Autodesk Fusion 360 part; units mm, degrees
sketch "Sketch1" plane through (0, 0, 0) normal (0, 0, 1) x (1, 0, 0)
  circle A0 centre (0, 0) radius 9.5
  line L0 (12, 5) -> (-12, 5)
  line L1 (-12, 5) -> (-12, -5)
  line L2 (-12, -5) -> (12, -5)
  line L3 (12, -5) -> (12, 5)
  line L4 (-12, -5) -> (-22, -5)
  line L5 (-22, -5) -> (-22, 5)
  line L6 (-22, 5) -> (-12, 5)
  line L7 (-12, 5) -> (-12, -5)
  line L8 (12, -5) -> (22, -5)
  line L9 (22, -5) -> (22, 5)
  line L10 (22, 5) -> (12, 5)
  line L11 (12, 5) -> (12, -5)
  circle A1 centre (17, 0) radius 1.825
  circle A2 centre (-17, 0) radius 1.825
  dimension "d1" = 19
  dimension "d2" = 5
  dimension "d3" = 5
  dimension "d4" = 12
  dimension "d19" = 24
  dimension "d20" = 3.65
  dimension "d21" = 3.65
extrude "Extrude1" add sketch "Sketch1" along normal blind 3 contours A0 L0 L2 L3 L11 | A0 L0 L1 L2 L7 makes body 1 at (-9.0078, 3.0183, 2) makes body 2 at (8.3, 4.6217, 2)
extrude "Extrude2" add sketch "Sketch1" along normal blind 13.5 contours A0 L0 L2 | A0 L0 | A0 L2 bodies 1 2
sketch "Sketch2" plane through (0, 0, 0) normal (0, 1, 0) x (1, 0, 0)
  line L0 (-9.5, -15) -> (9.5, -15)
  line L1 (9.5, -15) -> (9.5, 0)
  line L2 (9.5, 0) -> (-9.5, 0)
  line L3 (-9.5, 0) -> (-9.5, -15)
  line L4 (9.5, 0) -> (-9.5, 0)
  line L5 (-9.5, 0) -> (-9.5, -3)
  line L6 (-9.5, -3) -> (9.5, -3)
  line L7 (9.5, -3) -> (9.5, 0)
  line L8 (-9.5, -15) -> (9.5, -3)
  line L9 (-9.5, 0) -> (9.5, 0)
  dimension "d10" = 3
sphere "SpherePrimitive2" cut diameter 15.8 placed x (1, 0, 0) y (0, 0, -1) z (0, 1, 0) at (0, 0, 11) bodies 1
sketch "Sketch7" plane through (0, 0, 0) normal (1, 0, 0) x (0, 1, 0)
  line L0 (0, 3) -> (-3, 3)
  line L1 (-3, 3) -> (-3, 13.5)
  line L2 (-3, 13.5) -> (0, 13.5)
  line L3 (0, 13.5) -> (0, 3)
  line L4 (-5, 0) -> (-5, 3)
  line L5 (0, 15) -> (0, 0)
  line L6 (0, 3) -> (3, 3)
  line L7 (3, 3) -> (3, 13.5)
  line L8 (0, 13.5) -> (0, 3)
  line L9 (3, 13.5) -> (0, 13.5)
  line L10 (0, 13.5) -> (-5.5, 13.5)
  line L11 (-5.5, 13.5) -> (0, 3)
  line L12 (5.5, 13.5) -> (0, 3)
  line L13 (0, 13.5) -> (5.5, 13.5)
  dimension "d12" = 3
  dimension "d13" = 2
  dimension "d14" = 10.5
extrude "Extrude3" cut sketch "Sketch7" along normal blind 17 bodies 1
extrude "Extrude4" cut sketch "Sketch7" against normal blind 11 bodies 1
extrude "Extrude5" add sketch "Sketch1" along normal blind 1.5 contours L3 L8 L9 L10 L11 | L1 L4 L5 L6 L7 bodies 1
equation "d1 = 15 mm + 4 mm"
Geometry check sheet. Reference: the model listing, model coordinates, mm. A direction names the side the tool comes from. Round coordinates to 2 decimals unless told otherwise and drop trailing zeros. Order: outer loops, then holes, each group sorted by start corner. A loop starts at its lowest first (then second) coordinate and runs counter-clockwise, first axis right, second up. Notation, with made-up numbers: (-18.5, 21.25) - (26.5, 21.25) arc R17 ccw to (26.5, 34.25) - close; hole circle Ø2 at (36.25, -35.75). An arc over 180 degrees is marked (long way). Use a Markdown table: item, result. Add a question column.
1) Set-up check for faces 1 (the cylindrical face through (-0.17, 9.5, 6.66)), 2 (the flat face through (-13, 5, 1)), 3 (the flat face through (7.46, -4.27, 11.15)), 4 (the flat face through (-14, -5, 1)), 5 (the flat face through (13, -5, 1)): record each of +Z, -Z, +X, -X, +Y, -Y from which the full face is reachable in a straight line by a thin tool's end or side.
2) Section check B-B (y = 0). Record the cut outline in (x, z) (3 decimals).
3) Thickness scan on line 1 along Y through (x, z) = (17, 0.7) (3 decimals); line 2 along X through (y, z) = (-5.5, 4.5); line 3 along Z through (x, y) = (-5, -2.75). Record the ranges inside material, lowest first.
4) Section check D-D (y = 7.5). Record the cut outline in (x, z), then the cut area to 3 significant figures.
5) Section check C-C (z = 4.75). Record the cut outline in (x, y).
6) Gauge pin test, flat ends, axial feed: P1, Ø1.6, axis at y = -2, z = 2.5, coming from the +X side; P2, Ø3, axis at x = -15, y = -1, coming from the +Z side; P3, Ø5, axis at x = 1, z = 2, coming from the -Y side; P4, Ø0.9, axis at x = 17.5, z = 1, coming from the -Y side. Record the tip position at first contact, or that the pin passes through.
7) Mould release check, pull along Y, two halves, no side actions. Record for faces 6 (the flat face through (14, 5, 1)), 7 (the flat face through (0.1, 3, 3.3)), 8 (the flat face through (-0.1, -3, 3.3)), 9 (the cylindrical face through (0.17, -9.5, 6.66)): released by +Y, released by -Y, zero draft, split by the parting line, or undercut.
8) Section check A-A (x = 17). Record the cut outline in (y, z) (3 decimals), then the cut area to 4 significant figures.
Established:
| question | item | result |
|---|---|---|
| 1 | face 1 | +Z, +Y |
| 1 | face 2 | +Z, -Z, -X, +Y |
| 1 | face 3 | +Z, +X, -X |
| 1 | face 4 | +Z, -Z, -X, -Y |
| 1 | face 5 | +Z, -Z, +X, -Y |
| 2 | outline | (-22, 0) - (-18.825, 0) - (-18.825, 1.5) - (-22, 1.5) - close; (-15.175, 0) - (15.175, 0) - (15.175, 1.5) - (12, 1.5) - (12, 3) - (-12, 3) - (-12, 1.5) - (-15.175, 1.5) - close; (18.825, 0) - (22, 0) - (22, 1.5) - (18.825, 1.5) - close |
| 3 | line 1 | -5 to -1.825, 1.825 to 5 |
| 3 | line 2 | -7.75 to 7.75 |
| 3 | line 3 | 0 to 3 |
| 4 | outline | (-5.83, 0) - (5.83, 0) - (5.83, 13.5) - (-5.83, 13.5) - close; hole circle Ø4.96 at (0, 11) |
| 4 | area | 138 mm2 |
| 5 | outline | (-9.01, -3) arc R9.5 ccw to (9.01, -3) - (3.79, -3) arc R4.83 cw to (-3.79, -3) - close; (-9.01, 3) - (-3.79, 3) arc R4.83 cw to (3.79, 3) - (9.01, 3) arc R9.5 ccw to start |
| 6 | P1 | x = 12 |
| 6 | P2 | z = 1.5 |
| 6 | P3 | y = -9.5 |
| 6 | P4 | y = -5 |
| 7 | face 6 | released by +Y |
| 7 | face 7 | undercut |
| 7 | face 8 | undercut |
| 7 | face 9 | released by -Y |
| 8 | outline | (-5, 0) - (-1.825, 0) - (-1.825, 1.5) - (-5, 1.5) - close; (1.825, 0) - (5, 0) - (5, 1.5) - (1.825, 1.5) - close |
| 8 | area | 9.525 mm2 |
